Here's how the part is built. I have some questions about the finished solid (model axes, mm). A direction names the side the tool comes from. Round coordinates to 2 decimals unless told otherwise and drop trailing zeros. Write each loop counter-clockwise with the first axis right and the second up, starting at its lowest first coordinate (ties: lowest second). Pieces come first, ordered by that corner, then holes. Notation, with made-up numbers: (-1, 18.5) -> (43, 18.5) arc R30 ccw to (43, 57.5) -> close; hole circle Ø11 at (47.5, -14). An arc over 180 degrees is marked (long way). Answer in a Markdown table with one row per item.
from build123d import *

# Parameters (mm, degrees)
F0_R     = 10
F1_DEPTH = 300
F3_DEPTH = 15
F5_DEPTH = 14.142


# Not quite as in the source:
# - a feature of the source that left no trace in its solid (it failed there, or was rolled back) is left out


with BuildPart() as f1:
    # F0 (on Top) → F1 (new body)
    with BuildSketch(Plane.XY):
        Circle(F0_R)
    extrude(amount=F1_DEPTH)

    # F2 (on face) → F3 (join)
    with BuildSketch(Plane.XY.offset(300)):
        Polygon((10, 0), (10, 10), (0, 10), (-10, 10), (-10, 0), (-10, -10), (0, -10), (10, -10), align=None)
        Polygon((0, 10), (10, 10), (10, 0), (66.5685424949, 56.5685424949), (56.5685424949, 66.5685424949), align=None)
        Polygon((-10, 10), (0, 10), (-56.5685424949, 66.5685424949), (-66.5685424949, 56.5685424949), (-10, 0), align=None)
        Polygon((66.5685424949, -56.5685424949), (10, 0), (10, -10), (0, -10), (56.5685424949, -66.5685424949), align=None)
        Polygon((-10, -10), (-10, 0), (-66.5685424949, -56.5685424949), (-56.5685424949, -66.5685424949), (0, -10), align=None)
    extrude(amount=-F3_DEPTH)

    # F4 (on face) → F5 (join)
    with BuildSketch(Plane(origin=(5, -5, 0), x_dir=(0.7071067812, 0.7071067812, 0), z_dir=(0.7071067812, -0.7071067812, 0))):
        Polygon((129.2763065782, 257.7947612337), (87.0710678119, 300), (87.0710678119, 285), (114.2763065782, 257.7947612337), (114.2763065782, 242.7947612337), (129.2763065782, 242.7947612337), align=None)
        Polygon((119.3018365804, 225.5184724189), (129.2763065782, 242.7947612337), (114.2763065782, 242.7947612337), (104.3018365804, 225.5184724189), align=None)
    extrude(amount=-F5_DEPTH)

    # F6: F1 across plane


with BuildPart() as f1_1:
    add(f1.part)
    add(f1.part.mirror(Plane.XZ))

    # F7: F1 across plane


with BuildPart() as f1_2:
    add(f1_1.part)
    add(f1_1.part.mirror(Plane.YZ))


solid = f1_2.part
1) For pin 1 (22.5 mm diameter, centred on x = -80, y = 82.5, fed in from -Z); pin 2 (2 mm diameter, centred on x = 14.5, y = -11.5, fed in from -Z); pin 3 (10 mm diameter, centred on x = -71, y = -55, fed in from -Z), each with a flat end and sliding along its axis, tell me the tip position at first contact or that it passes through.
Response:
| item | result |
|---|---|
| pin 1 | stops at z = 225.52 |
| pin 2 | stops at z = 285 |
| pin 3 | stops at z = 280.33 |
2) I want a section at A-A, the plane x = 46.5. List the corners of the cut face in (y, z) for me.
Response:
| item | result |
|---|---|
| outline | (-56.5, 285) -> (-36.5, 285) -> (-36.5, 300) -> (-56.5, 300) -> close; (36.5, 285) -> (56.5, 285) -> (56.5, 300) -> (36.5, 300) -> close |
3) We'd pull the mould along X, two halves only. Please class faces 1 (the face through (-71.12, -70.98, 271.59)), 2 (the face through (-2.17, -9.76, 140.5)), 3 (the face through (87.906, 87.766, 234.036)): +X half, -X half, draft (parallel to the pull), parting line (faces both ways), or undercut.
Response:
| item | result |
|---|---|
| face 1 | undercut |
| face 2 | parting line |
| face 3 | +X half |
4) I want a section at C-C, the plane z = 110.5. List the corners of the cut face in (x, y) for me.
Response:
| item | result |
|---|---|
| outline | circle Ø20 at (0, 0) |
5) Which directions (+Z, -Z, +X, -X, +Y, -Y) give clear straight access to the entire face, cutting with the end or side of a thin tool? Please do faces 4 (the face through (-75, 85, 263)), 5 (the face through (71.12, -70.98, 271.59)), 6 (the face through (-75, -85, 263)).
Response:
| item | result |
|---|---|
| face 4 | +Z, -Z, +Y |
| face 5 | none |
| face 6 | +Z, -Z, -Y |
6) I want a section at D-D, the plane x = -62.5. List the corners of the cut face in (y, z) for me, and give its area (3 significant figures).
Response:
| item | result |
|---|---|
| outline | (-72.5, 276.61) -> (-60.64, 285) -> (-52.5, 285) -> (-52.5, 300) -> (-60.64, 300) -> (-72.5, 291.61) -> close; (52.5, 285) -> (60.64, 285) -> (72.5, 276.61) -> (72.5, 291.61) -> (60.64, 300) -> (52.5, 300) -> close |
| area | 600 mm^2 |
7) I want a section at B-B, the plane z = 232. List the corners of the cut face in (x, y) for me.
Response:
| item | result |
|---|---|
| outline | (-92.01, -82.01) -> (-82.01, -92.01) -> (-71.4, -81.4) -> (-81.4, -71.4) -> close; (-92.01, 82.01) -> (-81.4, 71.4) -> (-71.4, 81.4) -> (-82.01, 92.01) -> close; circle Ø20 at (0, 0); (71.4, -81.4) -> (82.01, -92.01) -> (92.01, -82.01) -> (81.4, -71.4) -> close; (71.4, 81.4) -> (81.4, 71.4) -> (92.01, 82.01) -> (82.01, 92.01) -> close |
8) I need wall thicknesses on line 1 (Z direction, x = 9.5, y = -13); line 2 (Y direction, x = 9, z = 157); line 3 (X direction, y = 75, z = 281.5). Which ranges of each line are inside material? Lowest first, please. Write a range as [from, to].
Response:
| item | result |
|---|---|
| line 1 | z = [285, 300] |
| line 2 | y = [-4.36, 4.36] |
| line 3 | x = [-74.3, -65], [65, 74.3] |
